```python
from build123d import *

# Parameters (mm, degrees)
EXTRUDE_1_DEPTH     = 80
CHAMFER_1_SIZE      = 5
SKETCH_2_R          = 1.55
CUT_EXTRUDE_1_DEPTH = 250
SKETCH_3_R          = 1.55
CUT_EXTRUDE_2_DEPTH = 106


with BuildPart() as part:
    # 草图1 → 拉伸-薄壁1 (new body)
    with BuildSketch(Plane.XY):
        Polygon((0, 0), (20, 0), (20, 65), (0, 65), (0, 61), (16, 61), (16, 4), (0, 4), align=None)
    extrude(amount=EXTRUDE_1_DEPTH)

    # 倒角1
    chamfer_1_edges = [part.edges().sort_by_distance(p)[0] for p in [
        (16, 4, 40),
        (16, 61, 40),
    ]]
    chamfer(chamfer_1_edges, length=CHAMFER_1_SIZE)

    # 草图2 → 切除-拉伸1 (cut, symmetric)
    with BuildSketch(Plane.XZ.offset(-61)):
        with Locations(Location((5.5, 12, 0), (0, 0, 90))):
            Circle(SKETCH_2_R)
        with Locations(Location((5.5, 68, 0), (0, 0, 90))):
            Circle(SKETCH_2_R)
        with Locations(Location((5.5, 33, 0), (0, 0, 90))):
            Circle(SKETCH_2_R)
        with Locations(Location((5.5, 47, 0), (0, 0, 90))):
            Circle(SKETCH_2_R)
    extrude(amount=CUT_EXTRUDE_1_DEPTH, both=True, mode=Mode.SUBTRACT)

    # 草图3 → 切除-拉伸2 (cut, through all)
    with BuildSketch(Plane(origin=(20, 0, 0), x_dir=(0, 0, -1), z_dir=(1, 0, 0))):
        with Locations((-40, 42.5)):
            Circle(SKETCH_3_R)
        with Locations((-32.928932188, 39.571067812)):
            Circle(SKETCH_3_R)
        with Locations((-30, 32.5)):
            Circle(SKETCH_3_R)
        with Locations((-32.928932188, 25.428932188)):
            Circle(SKETCH_3_R)
        with Locations((-40, 22.5)):
            Circle(SKETCH_3_R)
        with Locations((-47.071067812, 25.428932188)):
            Circle(SKETCH_3_R)
        with Locations((-50, 32.5)):
            Circle(SKETCH_3_R)
        with Locations((-47.071067812, 39.571067812)):
            Circle(SKETCH_3_R)
    extrude(amount=-CUT_EXTRUDE_2_DEPTH, mode=Mode.SUBTRACT)


solid = part.part
```
Source: CAD feature listing. Evaluate the final solid. Frame: model axes, mm. A direction names the side the tool comes from. Give positions to 0.01 mm unless a question says otherwise; leave off trailing zeros. Loops run counter-clockwise (first coordinate to the right, second up) from the corner with the lowest first, then second, coordinate; pieces in that order, holes last. Notation, with made-up numbers: (43, 35.5) - (94, 35.5) arc R10 cw to (94, 53.5) - close; hole circle Ø4 at (77.25, 12.5). An arc over 180 degrees is marked (long way). Use CSV: the item, a comma, the result in double quotes. Start each with the question number.
1. Pin query (flat end, axial travel): pin 1 (3 mm diameter, centred on x = 5.5, z = 47, fed in from +Y); pin 2 (12 mm diameter, centred on x = 13, y = 28, fed in from +Z). Return the tip coordinate at first contact, or that it passes through.
2. Section D-D (z = 12). Output: boundary loops of the cut face in (x, y).
3. Reachability of faces 5 (the flat face through (14, 58, 39)), 6 (the cylindrical face through (5.034, 62.972, 69.478)) from +Z, -Z, +X, -X, +Y, -Y: full face, straight path, thin tool, end or side. Return the list, or none.
4. Section A-A (y = 32.5). Output: boundary loops of the cut face in (x, z).
5. Draft query along Y for faces 1 (the flat face through (10, 0, 39)), 2 (the cylindrical face through (18.028, 32.966, 28.522)), 3 (the cylindrical face through (5.034, 1.972, 48.478)), 4 (the cylindrical face through (18.03, 40.88, 32.1)). Return one class per face: +Y half, -Y half, draft (parallel to the pull), parting line (faces both ways), or undercut.
6. Section B-B (z = 50). Output: boundary loops of the cut face in (x, y), then the cut area to 3 significant figures.
7. Ray query, L1, parallel to Z at x = 5.5, y = 63.15; L2, parallel to Y at x = 18.6, z = 40; L3, parallel to Y at x = 7.25, z = 76.5. Return the intervals inside material, ascending.
8. Section C-C (y = 42.5). Output: boundary loops of the cut face in (x, z), then the cut area to 3 significant figures.
Response:
1,pin 1,"through"
1,pin 2,"z = 80"
2,outline,"(0, 0) - (3.95, 0) - (3.95, 4) - (0, 4) - close; (0, 61) - (3.95, 61) - (3.95, 65) - (0, 65) - close; (7.05, 0) - (20, 0) - (20, 65) - (7.05, 65) - (7.05, 61) - (11, 61) - (16, 56) - (16, 9) - (11, 4) - (7.05, 4) - close"
3,face 5,"+Z, -Z, -X"
3,face 6,"+Y, -Y"
4,outline,"(16, 0) - (20, 0) - (20, 28.45) - (16, 28.45) - close; (16, 31.55) - (20, 31.55) - (20, 48.45) - (16, 48.45) - close; (16, 51.55) - (20, 51.55) - (20, 80) - (16, 80) - close"
5,face 1,"-Y half"
5,face 2,"undercut"
5,face 3,"draft"
5,face 4,"undercut"
6,outline,"(0, 0) - (20, 0) - (20, 30.95) - (16, 30.95) - (16, 9) - (11, 4) - (0, 4) - close; (0, 61) - (11, 61) - (16, 56) - (16, 34.05) - (20, 34.05) - (20, 65) - (0, 65) - close"
6,area,"401 mm²"
7,L1,"0 to 10.45, 13.55 to 31.45, 34.55 to 45.45, 48.55 to 66.45, 69.55 to 80"
7,L2,"0 to 20.95, 24.05 to 40.95, 44.05 to 65"
7,L3,"0 to 4, 61 to 65"
8,outline,"(16, 0) - (20, 0) - (20, 38.45) - (16, 38.45) - close; (16, 41.55) - (20, 41.55) - (20, 80) - (16, 80) - close"
8,area,"308 mm²"
